Model file for the job. Use its own axes, mm. Face numbers are marked on the shaded views. A direction names the side the tool comes from. Coordinates: 2 decimals unless noted, no trailing zeros. Return JSON: item names as keys, results as strings. Group by question number.
1) Pull direction Z, two halves, no side cores. Call the marked faces 3, 4, 5 and 6: +Z half, -Z half, draft (parallel to the pull), parting line (faces both ways), or undercut.
2) Flat gauge pins, fed straight in: pin 1 (2 mm diameter, centred on x = 11.5, z = -0.5, fed in from -Y); pin 2 (3 mm diameter, centred on x = 12.5, y = 0, fed in from -Z). Where does each tip first touch, or does it go through?
3) Probe line 1 (Z direction, x = 6.75, y = 0.1); line 2 (X direction, y = -1.5, z = -1.7). List the from-to ranges inside material, lowest first.
4) Which spindle directions (+Z, -Z, +X, -X, +Y, -Y) get a long thin tool onto all of the face, cutting with end or side? Do the marked faces 1 and 2. Say none if no direction does.
from build123d import *

# Parameters (mm, degrees)
FILLET1_R       = 0.1
FILLET2_R       = 0.3
HEX_2_DEPTH     = 1.3
THDSCHPAT_COUNT = 29
THDSCHPAT_PITCH = 0.5


with BuildPart() as part:
    # BodySke → Base-Revolve (revolve)
    with BuildSketch(Plane.XY, mode=Mode.PRIVATE) as base_revolve_sk:
        Polygon((0, 0), (0, 2.75), (3, 2.75), (3, 1.5), (18.7195, 1.5), (19, 1.2195), (19, 0), align=None)
    revolve(base_revolve_sk.sketch.rotate(Axis((-31.75, 0, 0), (1, 0, 0)), 90), axis=Axis((-31.75, 0, 0), (1, 0, 0)))  # turned: the seam where the file's is

    # Fillet1
    fillet1_edges = [part.edges().sort_by_distance(p)[0] for p in [
        (3, 0, -1.5),
    ]]
    fillet(fillet1_edges, radius=FILLET1_R)

    # Fillet2
    fillet2_edges = [part.edges().sort_by_distance(p)[0] for p in [
        (0, 0, -2.75),
    ]]
    fillet(fillet2_edges, radius=FILLET2_R)

    # Sketch2 → Hex-PreBroach (revolve, cut)
    with BuildSketch(Plane.XY, mode=Mode.PRIVATE) as hex_prebroach_sk:
        Polygon((0, 1.26), (1.3, 1.26), (2.027461339, 0), (0, 0), align=None)
    revolve(hex_prebroach_sk.sketch.rotate(Axis((0, 0, 0), (1, 0, 0)), 90), axis=Axis((0, 0, 0), (1, 0, 0)), mode=Mode.SUBTRACT)  # turned: the seam where the file's is

    # Sketch3 → Hex 2 (cut)
    with BuildSketch(Plane(origin=(0, 0, 0), x_dir=(0, 0.5, 0.866025404), z_dir=(-1, 0, 0))):
        Polygon((0.727461339, 1.26), (-0.727461339, 1.26), (-1.454922678, 0), (-0.727461339, -1.26), (0.727461339, -1.26), (1.454922678, 0), align=None)
    extrude(amount=-HEX_2_DEPTH, mode=Mode.SUBTRACT)

    # ThdSchSke → ThreadSchematic (revolve, cut)
    with BuildSketch(Plane.XY, mode=Mode.PRIVATE) as threadschematic_sk:
        Polygon((4.5, -1.2195), (4.303591786, -1.5), (4.303591786, -1.875), (4.696408214, -1.875), (4.696408214, -1.5), align=None)
    threadschematic = revolve(threadschematic_sk.sketch.rotate(Axis((-3.175, 0, 0), (1, 0, 0)), 270), axis=Axis((-3.175, 0, 0), (1, 0, 0)), mode=Mode.SUBTRACT)  # turned: the seam where the file's is

    # ThdSchPat: ThreadSchematic ×29
    with Locations(*[(i * THDSCHPAT_PITCH, 0, 0) for i in range(1, THDSCHPAT_COUNT)]):
        add(threadschematic, mode=Mode.SUBTRACT)


solid = part.part
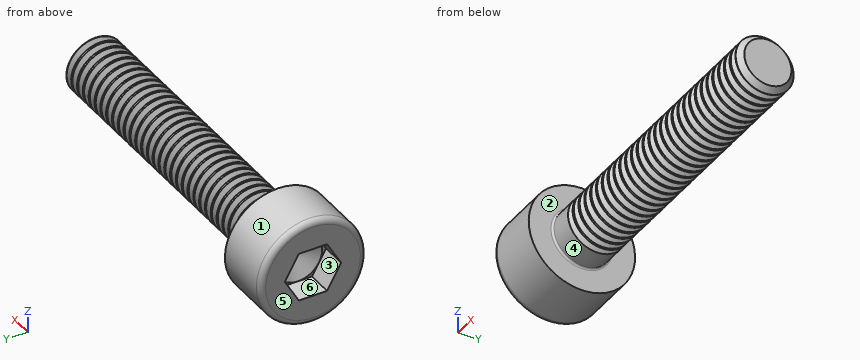
Answers below:
{
 "1": {"face 3": "undercut", "face 4": "parting line", "face 5": "draft", "face 6": "undercut"},
 "2": {"pin 1": "stops at y = -1.5", "pin 2": "stops at z = -1.5"},
 "3": {"line 1": "z = -1.5 to 1.5", "line 2": "x = 0 to 3"},
 "4": {"face 1": "+X, -X", "face 2": "+X"}
}
